Autodesk Inventor part; units mm, degrees
ref_plane "YZ Plane" through (0, 0, 0) normal (1, 0, 0) x (0, 1, 0)
ref_plane "XZ Plane" through (0, 0, 0) normal (0, 1, 0) x (-1, 0, 0)
ref_plane "XY Plane" through (0, 0, 0) normal (0, 0, 1) x (1, 0, 0)
sketch "Sketch1" plane through (0, 0, 0) normal (0, 1, 0) x (-1, 0, 0)
  circle A0 centre (-32.475, -32.475) radius 3.3
  circle A1 centre (-32.475, -32.475) radius 7.5
  line L0 (25, 0) -> (0, 0)
  line L1 (0, 0) -> (0, -15)
  line L2 (0, -15) -> (25, -15)
  line L3 (25, -15) -> (25, 0)
  line L4 (0, 20) -> (-29, 20)
  line L5 (-29, 20) -> (-29, 0)
  line L6 (-29, 0) -> (0, 0)
  line L7 (0, 0) -> (0, 20)
  line L8 (0, 0) -> (-36.8411, -26.3768)
  line L9 (0, -15) -> (-27.6522, -38.2187)
  line L10 (-29, 0) -> (-39.5499, -29.9858)
  line L11 (0, 0) -> (-55.6524, 0) construction
  line L12 (-55.6524, 0) -> (-55.6524, -63.0935) construction
  line L13 (-55.6524, -63.0935) -> (0, -63.0935) construction
  line L14 (0, -63.0935) -> (0, 0) construction
  dimension "d0" = 6.6
  dimension "d1" = 32.475
  dimension "d2" = 32.475
  dimension "d3" = 15
  dimension "d4" = 25
  dimension "d6" = 15
  dimension "d7" = 29
  dimension "d8" = 20
extrude "Extrusion1" add sketch "Sketch1" along normal blind 12 contours A1 | A1 L8 L1 L9 | A1 L10 L6 L8 | L0 L3 L2 L1
sketch "Sketch2" plane through (0, 12, 0) normal (0, 1, 0) x (1, 0, 0)
  circle A0 centre (32.475, 32.475) radius 3.3
  circle A1 centre (32.475, 32.475) radius 10
  line L0 (-25, 15) -> (-25, 0)
  line L1 (-25, 0) -> (29, 0)
  line L2 (29, 0) -> (39.5499, 29.9858)
  arc A2 (39.5499, 29.9858) -> (27.6522, 38.2187) centre (32.475, 32.475) ccw
  line L3 (27.6522, 38.2187) -> (0, 15)
  line L4 (0, 15) -> (-25, 15)
  circle A3 centre (32.475, 32.475) radius 3.3
  line L5 (-25, 15) -> (-25, 0)
  line L6 (-25, 12) -> (0, 12)
  line L7 (0, 12) -> (0, 3)
  line L8 (0, 3) -> (-25, 3)
  line L9 (-25, 3) -> (-25, 12)
  line L10 (27.6522, 38.2187) -> (0, 15)
  line L11 (0, 15) -> (0, 0)
  line L12 (29, 0) -> (39.5499, 29.9858)
  line L13 (0, 0) -> (30.0555, 0)
  line L14 (30.0555, 0) -> (30.0555, 3)
  line L15 (30.0555, 3) -> (0, 3)
  line L16 (0, 3) -> (0, 0)
  point P0 (37.3547, 23.7464)
  point P1 (22.5867, 33.9654)
  point P2 (-25, 7.5)
  point P3 (-25, 3)
  dimension "d11" = 20
  dimension "d14" = 9
extrude "Extrusion2" cut sketch "Sketch2" against normal blind 3 contours A1 L2 L15 L7 L11 L3 | L14 L13 L2 | L7 L8 L0 L6
sketch "Sketch6" plane through (0, 0, 0) normal (0, -1, 0) x (1, 0, 0)
  line L0 (0, -15) -> (-25, -15)
  line L1 (-25, 0) -> (29, 0)
  line L2 (-22, -15) -> (-19, -15)
  line L3 (-19, -15) -> (-19, 0)
  line L4 (-19, 0) -> (-22, 0)
  line L5 (-22, 0) -> (-22, -15)
  line L6 (-6, -15) -> (-3, -15)
  line L7 (-3, -15) -> (-3, 0)
  line L8 (-3, 0) -> (-6, 0)
  line L9 (-6, 0) -> (-6, -15)
  line L10 (-25, -15) -> (-25, 0)
  point P0 (0, 0)
  point P1 (-2, 0)
  point P2 (-3, 0)
  point P3 (-22, 0)
  point P4 (-19, -15)
  dimension "d31" = 3
  dimension "d32" = 3
  dimension "d33" = 3
  dimension "d34" = 3
extrude "Extrusion6" cut sketch "Sketch6" against normal blind 2 contours L0 L9 L1 L7 | L0 L5 L1 L3
chamfer "Chamfer1" distance 1.75 angle 45 2 edges at (35.775, 12, -32.475) (35.775, 0, -32.475)
fillet "Fillet1" radius 2 3 edges at (2.5277, 12, -3) (-12.5, 12, -12) (26.7848, 12, -24.2518)
equation "\"d2\" = d1"
properties part number "Strain Relief"
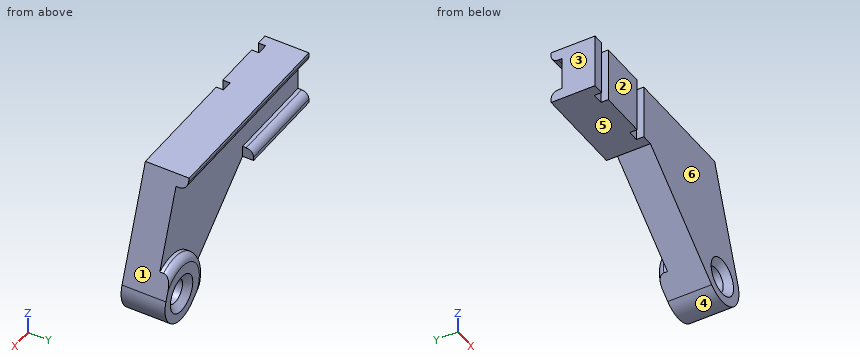
Here's how the part is built. I have some questions about the finished solid (model axes, mm). Face numbers are marked on the shaded views. A direction names the side the tool comes from. Round coordinates to 2 decimals unless told otherwise and drop trailing zeros. Loops run counter-clockwise (first coordinate to the right, second up) from the corner with the lowest first, then second, coordinate; pieces in that order, holes last. Notation, with made-up numbers: (26, 31.5) -> (51, 31.5) arc R19 cw to (51, 38.5) -> close; hole circle Ø3 at (-31.5, 78.5). An arc over 180 degrees is marked (long way). Answer as CSV lines item,"result". Start each with the question number.
1. Imagine slicing it at B-B on y = 4.25. Write out the boundary of the cut face in (x, z) (3 decimals), plus the area to 3 significant figures.
2. For the marked faces 5 and 6, which set-ups out of +Z, -Z, +X, -X, +Y, -Y let a thin tool reach every point of the face, with its end or its side?
3. If we mould it in two halves opening along X, with no side actions, what happens to the marked faces 1, 2, 3 and 4? For each: pulls with the +X half, pulls with the -X half, needs draft (parallel to the pull), parting line crosses it, or undercut.
4. I'm going to push flat-ended pins straight in: P1, Ø9.5, axis at x = -8, z = -17, coming from the +Y side; P2, Ø1.5, axis at x = -21, z = -5.5, coming from the -Y side; P3, Ø2.5, axis at y = 10.5, z = -13.5, coming from the +X side; P4, Ø6, axis at y = 8, z = -25, coming from the -X side. Where does each tip first touch, or does it pass through?
5. Imagine slicing it at A-A on x = -4. Write out the boundary of the cut face in (y, z), plus the area to 3 significant figures.
6. Imagine slicing it at D-D on x = -14. Write out the boundary of the cut face in (y, z), plus the area to 3 significant figures.
7. Imagine slicing it at C-C on z = -8.5. Write out the boundary of the cut face in (x, y), plus the area to 3 significant figures.
8. I need wall thicknesses on probe 1 along Y at (x, z) = (-11, -6.5); probe 2 along Z at (x, y) = (-9.5, 1); probe 3 along X at (y, z) = (11, -31.5). Which ranges of each line are inside material? Lowest first, please. Write a range as from..to.
Solution:
1,outline,"(-25, -15) -> (0, -15) -> (27.652, -38.219) arc R7.5 ccw to (39.55, -29.986) -> (29, 0) -> (-25, 0) -> close; hole circle Ø6.6 at (32.475, -32.475)"
1,area,"1,380 mm²"
2,face 5,"-Z, -X, +Y, -Y"
2,face 6,"+Z, -Z, +X, -X, -Y"
3,face 1,"pulls with the +X half"
3,face 2,"needs draft"
3,face 3,"pulls with the -X half"
3,face 4,"parting line crosses it"
4,P1,"y = 12"
4,P2,"y = 2"
4,P3,"x = 0"
4,P4,"x = 8.34"
5,outline,"(2, -15) -> (12, -15) -> (12, -14) arc R2 ccw to (10, -12) -> (9, -12) -> (9, -3) -> (10, -3) arc R2 ccw to (12, -1) -> (12, 0) -> (2, 0) -> close"
5,area,"121 mm²"
6,outline,"(0, -15) -> (12, -15) -> (12, -14) arc R2 ccw to (10, -12) -> (9, -12) -> (9, -3) -> (10, -3) arc R2 ccw to (12, -1) -> (12, 0) -> (0, 0) -> close"
6,area,"151 mm²"
7,outline,"(-25, 0) -> (-22, 0) -> (-22, 2) -> (-19, 2) -> (-19, 0) -> (-6, 0) -> (-6, 2) -> (-3, 2) -> (-3, 0) -> (31.99, 0) -> (31.99, 9) -> (-25, 9) -> close"
7,area,"501 mm²"
8,probe 1,"0..9"
8,probe 2,"-15..0"
8,probe 3,"22.79..28.54, 36.41..39.91"
